Design review of the part built by this model. Coordinates are the model's own, in mm. A direction names the side the tool comes from. Give positions to 0.01 mm unless a question says otherwise; leave off trailing zeros. Order: outer loops, then holes, each group sorted by start corner. A loop starts at its lowest first (then second) coordinate and runs counter-clockwise, first axis right, second up. Notation, with made-up numbers: (87, 9.5) -> (100, 9.5) arc R37 ccw to (100, 46.5) -> close; hole circle Ø3 at (26.5, 69.25). An arc over 180 degrees is marked (long way). One line per item, written item: value. Start each with the question number.
1) Consider section A-A (x = -12.7). State the section outline as (y, z) points (3 decimals), plus the area to 3 significant figures.
2) Tool access review of faces 4 (the face through (10.34, -1.93, -0.77)), 5 (the face through (0, 9.525, -19)): name each direction out of +Z, -Z, +X, -X, +Y, -Y from which nothing blocks a thin tool from reaching the whole face with its end or side.
3) Consider section C-C (x = -8). State the section outline as (y, z) points (3 decimals), plus the area to 3 significant figures.
4) Wall thickness on line 1 along Z through (x, y) = (7.5, -6); line 2 along Y through (x, z) = (15, -12.5) (3 decimals); line 3 along Y through (x, z) = (12.7, -0.7) (3 decimals): over which ranges is each line inside the solid? List them lowest first. Write a range as from..to.
5) The part is to be moulded in two halves that separate along Z. For faces 1 (the face through (-9.677, 10.295, -31.103)), 2 (the face through (0, 11.044, -18)), 3 (the face through (0, -1, -1.519)), say which applies: released by +Z, released by -Z, zero draft, split by the parting line, or undercut.
6) For pin 1 (8.5 mm diameter, centred on x = -1, y = -5, fed in from -Z); pin 2 (8 mm diameter, centred on x = -6, z = -29, fed in from -Y) (3 decimals), all flat-tipped, find the tip position at first contact; note any pin that passes through.
7) Consider section B-B (y = -4). State the section outline as (x, z) points, plus the area to 3 significant figures.
from build123d import *

# Parameters (mm, degrees)
SKETCH7_W                    = 38.1
SKETCH7_H                    = 19.05
BASE_FLANGE1_DEPTH           = 1.51892
EDGE_FLANGE1_STRIP_W         = 9.88568
EDGE_FLANGE1_STRIP_H         = 1.51892
EDGE_FLANGE1_STRIP_CUT_DEPTH = 38.1
EDGE_FLANGE1_DEPTH           = 38.1
F_10_CLEARANCE_HOLE1_D       = 5.1054
F_10_CLEARANCE_HOLE2_D       = 5.1054
SKETCH24_W                   = 38.1
SKETCH24_H                   = 12.2555
CUT_EXTRUDE1_DEPTH           = 54.281766168


# Sheet-metal steps are written as plain solids
with BuildPart() as part:
    # Sketch7 → Base-Flange1 (new body)
    with BuildSketch(Plane.XY):
        Rectangle(SKETCH7_W, SKETCH7_H)
    extrude(amount=-BASE_FLANGE1_DEPTH)

    # Edge-Flange1 strip (across the edge) → Edge-Flange1 strip cut (cut)
    with BuildSketch(Plane(origin=(-19.05, 9.525, -1.51892), x_dir=(0, -1, 0), z_dir=(1, 0, 0))):
        with Locations((-3.03784, -0.75946)):
            Rectangle(EDGE_FLANGE1_STRIP_W, EDGE_FLANGE1_STRIP_H)
    extrude(amount=EDGE_FLANGE1_STRIP_CUT_DEPTH, mode=Mode.SUBTRACT)

    # Edge-Flange1 section (across the edge) → Edge-Flange1 (add)
    with BuildSketch(Plane(origin=(-19.05, 9.525, -1.51892), x_dir=(0, -1, 0), z_dir=(1, 0, 0))):
        with BuildLine():
            Line((-1.51892, 1.905), (-1.51892, 44.45))
            Line((-1.51892, 44.45), (0, 44.45))
            Line((0, 44.45), (0, 1.905))
            ThreePointArc((0, 1.905), (0.557961582, 0.557961582), (1.905, 0))
            Line((1.905, 0), (1.905, -1.51892))
            ThreePointArc((1.905, -1.51892), (-0.51607705, -0.51607705), (-1.51892, 1.905))
        make_face()
    extrude(amount=EDGE_FLANGE1_DEPTH)

    # #10 Clearance Hole1 (through all)
    with Locations(Plane.XY):
        with Locations((-12.7, -0.9525), (12.7, -0.9525)):
            Hole(F_10_CLEARANCE_HOLE1_D / 2)

    # #10 Clearance Hole2 (through all)
    with Locations(Plane(origin=(0, 9.525, 0), x_dir=(-1, 0, 0), z_dir=(0, -1, 0))):
        with Locations((-11.049, 18.53692), (11.049, 28.95092)):
            Hole(F_10_CLEARANCE_HOLE2_D / 2)

    # Sketch24 → Cut-Extrude1 (cut, through all)
    with BuildSketch(Plane.XZ.offset(-9.525)):
        with Locations((0, -39.84117)):
            Rectangle(SKETCH24_W, SKETCH24_H)
    extrude(amount=-CUT_EXTRUDE1_DEPTH, mode=Mode.SUBTRACT)


solid = part.part
Checked values:
1. outline: (-9.525, -1.519) -> (-3.505, -1.519) -> (-3.505, 0) -> (-9.525, 0) -> close; (1.6, -1.519) -> (7.62, -1.519) arc R1.905 cw to (9.525, -3.424) -> (9.525, -27.004) -> (11.044, -27.004) -> (11.044, -3.424) arc R3.424 ccw to (7.62, 0) -> (1.6, 0) -> close; (9.525, -33.713) -> (11.044, -33.713) -> (11.044, -30.898) -> (9.525, -30.898) -> close
1. area: 64.7 mm^2
2. face 4: +Z, -Z
2. face 5: -Z, +X, -X, -Y
3. outline: (-9.525, -1.519) -> (7.62, -1.519) arc R1.905 cw to (9.525, -3.424) -> (9.525, -33.713) -> (11.044, -33.713) -> (11.044, -3.424) arc R3.424 ccw to (7.62, 0) -> (-9.525, 0) -> close
3. area: 78.4 mm^2
4. line 1: z = -1.52..0
4. line 2: y = 9.525..11.044
4. line 3: y = -9.525..-3.505, 1.6..9.694
5. face 1: undercut
5. face 2: zero draft
5. face 3: released by -Z
6. pin 1: stops at z = -1.52
6. pin 2: stops at y = 9.525
7. outline: (-19.05, -1.52) -> (19.05, -1.52) -> (19.05, 0) -> (-19.05, 0) -> close
7. area: 57.9 mm^2
